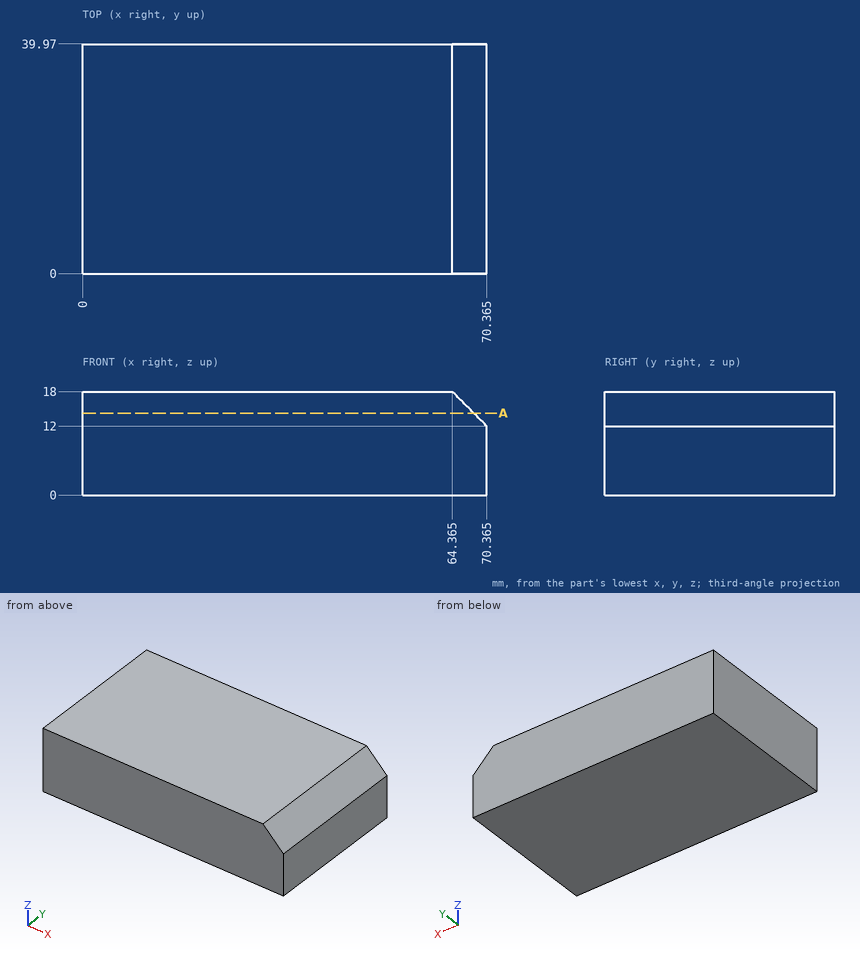
Drawing for the job (mm, zero at the part's lowest x, y, z). Round coordinates to 2 decimals unless told otherwise and drop trailing zeros. Write each loop counter-clockwise with the first axis right and the second up, starting at its lowest first coordinate (ties: lowest second). Pieces come first, ordered by that corner, then holes. Notation, with made-up numbers: M 26.25,83 L 76.25,83 A22 cw 76.25,106 Z; hole C 8,81.5 d8. An arc over 180 degrees is marked long. One line per question, with ' | ' between items.
1. Pin check, flat tip, straight feed: pin 1 Ø2 at (y, z) = (32.5, 13.5) entering from +X (1 decimal). Stop position of the tip, or through.
Working result:
pin 1: x = 69.9
2. Probe L1, parallel to X at y = 12, z = 13 (1 decimal); L2, parallel to X at y = 23.5, z = 15 (1 decimal); L3, parallel to Z at x = 66, y = 20 (1 decimal). List the from-to ranges inside material, lowest first. Write a range as from..to.
Working result:
L1: 0..69.4 | L2: 0..67.4 | L3: 0..16.4
3. Cut at A-A on z = 14.25. Write the cut outline in (x, y) (1 decimal), and give its area (3 significant figures).
Working result:
outline: M 0,0 L 68.1,0 L 68.1,40 L 0,40 Z | area: 2,720 mm2
